Autodesk Inventor part; units mm, degrees
ref_plane "YZ Plane" through (0, 0, 0) normal (1, 0, 0) x (0, 1, 0)
ref_plane "XZ Plane" through (0, 0, 0) normal (0, 1, 0) x (-1, 0, 0)
ref_plane "XY Plane" through (0, 0, 0) normal (0, 0, 1) x (1, 0, 0)
sketch "Sketch1" plane through (0, 0, 0) normal (0, 1, 0) x (-1, 0, 0)
  line L0 (-1.99, -2.7996) -> (-2.9, -2.7996)
  line L1 (-2.9, -2.7996) -> (-2.3804, -1.8996)
  line L2 (-2.3804, -1.8996) -> (-1.275, -1.8996)
  line L3 (-1.275, -1.8996) -> (-1.275, -2.7996)
  line L4 (-1.275, -2.7996) -> (-1.225, -2.7996)
  line L5 (-1.225, -2.7996) -> (-1.225, 3.8354)
  line L6 (-1.225, 3.8354) -> (-2.8, 3.8354)
  line L7 (-2.8, 3.8354) -> (-3.2, 2.8354)
  line L8 (-3.2, 2.8354) -> (-4, 2.8354)
  arc A0 (-2.5786, 4.3289) -> (-4, 2.8354) centre (-2.1332, 2.4819) ccw
  arc A1 (0, 4.6354) -> (-2.5786, 4.3289) centre (0, -6.3646) ccw
  line L9 (-1.99, -8.7996) -> (-1.99, -2.7996)
  spline S0 degree 3 poles (-1.99, -8.7996) (-1.99, -8.9227) (-1.9611, -9.0675) (-1.8666, -9.2952) (-1.7841, -9.4182) (-1.6089, -9.5929) (-1.4849, -9.6753) (-1.2538, -9.7706) (-1.1056, -9.7996) (-0.9798, -9.7996) knots 0.751438 0.751438 0.751438 0.751438 0.788362 0.788362 0.82538 0.82538 0.862606 0.862606 0.900353 0.900353 0.900353 0.900353
  line L10 (0, 4.6354) -> (0, -9.7996)
  line L11 (0, -9.7996) -> (-0.9798, -9.7996)
  point P0 (0, 0)
  point P1 (0, 0)
revolve "Revolution1" add sketch "Sketch1" angle 360 about axis through (0, 0, 4.6354) along (0, 0, -1)
sketch "Sketch2" plane through (0, 0, -9.7996) normal (0, 0, -1) x (-1, 0, 0)
  line L0 (0, 0.2829) -> (-1.2586, 1.5414)
  arc A0 (0.5514, 0.8343) -> (-0.5514, 0.8343) centre (0, 0) ccw
  line L1 (1.2586, 1.5414) -> (0, 0.2829)
  line L2 (0, -0.2829) -> (1.2585, -1.5414)
  arc A1 (-0.5514, -0.8343) -> (0.5514, -0.8343) centre (0, 0) ccw
  line L3 (-1.2586, -1.5414) -> (0, -0.2829)
  line L4 (0.2829, 0) -> (1.5414, 1.2586)
  arc A2 (0.8343, -0.5514) -> (0.8343, 0.5514) centre (0, 0) ccw
  line L5 (1.5414, -1.2585) -> (0.2829, 0)
  arc A3 (-0.8343, 0.5514) -> (-0.8343, -0.5514) centre (0, 0) ccw
  line L6 (-0.2829, 0) -> (-1.5414, -1.2585)
  line L7 (-1.5414, 1.2586) -> (-0.2829, 0)
  arc A4 (-1.2657, -1.5485) -> (1.2657, -1.5485) centre (0, 0) ccw
  circle A5 centre (0, 0) radius 1.99
  point P0 (0, 0)
  point P1 (0, 0)
  point P2 (-1.99, 0)
extrude "Extrusion1" cut sketch "Sketch2" against normal blind 3 contours L1 A5 L4 L5 L2 L3 L6 L7 L0
properties part number "11-6002" material "Polystyrene, High Impact"
Geometry: final body of the model. Coordinates: model frame, mm. A direction names the side the tool comes from. Coordinates: 2 decimals unless noted, no trailing zeros. Order: outer loops, then holes, each group sorted by start corner. A loop starts at its lowest first (then second) coordinate and runs counter-clockwise, first axis right, second up.
(1) Material intervals for probe 1 along X at (y, z) = (-0.75, -7.25); probe 2 along Y at (x, z) = (1, -7.25); probe 3 along Z at (x, y) = (-1.25, -0.75), sorted ascending.
(2) Section query A-A (z = -3.25). Return the cut outline in (x, y), plus the area to 3 significant figures.
(3) Draft query along Y for faces 3 (the face through (1.84, -0.76, -5.76)), 4 (the face through (-2, -3, 2.835)), 5 (the face through (-0.62, -0.903, -8.321)). Return one class per face: pulls with the +Y half, pulls with the -Y half, needs draft (parallel to the pull), parting line crosses it, or undercut.
(4) Section query B-B (z = -0.5). Return the cut outline in (x, y) (3 decimals).
(5) First-contact query: pin 1 (4 mm diameter, centred on x = 2.5, y = 2.5, fed in from -Z); pin 2 (4 mm diameter, centred on x = -0.5, z = -4, fed in from -Y); pin 3 (2 mm diameter, centred on x = 2, z = -7.5, fed in from +Y). Flat tips, straight axial feed; report the tip coordinate or a pass-through.
(6) Access query for faces 1 (the face through (-0.266, -1.196, 0.564)), 2 (the face through (-0.921, -0.638, -8.321)). Directions: +Z, -Z, +X, -X, +Y, -Y. A direction counts if a zero-diameter tool reaches every point of the face in a straight line with its end or side. Return the directions, or none.
Solution:
1. probe 1: x = -1.84 to -1.03, -0.47 to 0.47, 1.03 to 1.84
1. probe 2: y = -1.72 to -1.28, -0.72 to 0.72, 1.28 to 1.72
1. probe 3: z = -9.68 to -1.9, 3.84 to 4.54
2. outline: circle Ø3.98 at (0, 0)
2. area: 12.4 mm2
3. face 3: parting line crosses it
3. face 4: needs draft
3. face 5: undercut
4. outline: circle Ø2.45 at (0, 0)
5. pin 1: stops at z = -9.62
5. pin 2: stops at y = -2.9
5. pin 3: stops at y = 1.72
6. face 1: none
6. face 2: -Z
